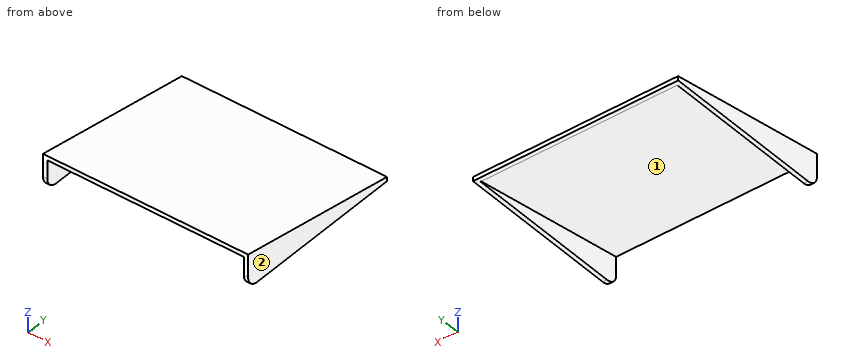
from build123d import *

# Parameters (mm, degrees)
F1_DEPTH = 914.4
F2_T     = -19.05


with BuildPart() as f1:
    # F0 (on Right) → F1 (new body)
    with BuildSketch(Plane.YZ):
        with BuildLine():
            Line((-889, 152.4), (-889, 50.8))
            ThreePointArc((-889, 50.8), (-874.121024, 14.878976), (-838.2, 0))
            Line((-838.2, 0), (-111.125, 0))
            Line((-111.125, 0), (-111.125, 19.05))
            Line((-111.125, 19.05), (-889, 152.4))
        make_face()
    extrude(amount=F1_DEPTH)

    # F2
    f2_openings = [f1.faces().sort_by_distance(p)[0] for p in [
        (457.2, -474.6625, 0),
        (457.2, -874.121024, 14.878976),
        (457.2, -889, 101.6),
    ]]
    offset(amount=F2_T, openings=f2_openings)


solid = f1.part
Geometry check sheet. Reference: the model listing, model coordinates, mm. Face numbers are marked on the shaded views. A direction names the side the tool comes from. Give positions to 0.01 mm unless a question says otherwise; leave off trailing zeros. Loops run counter-clockwise (first coordinate to the right, second up) from the corner with the lowest first, then second, coordinate; pieces in that order, holes last. Notation, with made-up numbers: M 79,1 L 90,1 A15 ccw 90,28 Z; hole C 17,72.25 d8. An arc over 180 degrees is marked long. Write each question's results on one line, items separated by ' | '.
1) Tool access check on the marked faces 1 and 2. Record the directions out of +Z, -Z, +X, -X, +Y, -Y that give a thin tool (end or side, any length) a straight path to the whole face; none if there is none.
Answers follow:
face 1: -Z, -Y | face 2: +Z, -Z, +X, +Y, -Y
2) Section check A-A, the plane y = -773.5. Record the boundary of the cut face in (x, z).
Answers follow:
outline: M 0,0 L 19.05,0 L 19.05,113.27 L 895.35,113.27 L 895.35,0 L 914.4,0 L 914.4,132.6 L 0,132.6 Z
3) Thickness scan on line 1 (X direction, y = -640, z = 16); line 2 (Z direction, x = 411, y = -845); line 3 (Z direction, x = 141, y = -790.5). Record the ranges inside material, lowest first.
Answers follow:
line 1: 0 to 19.05, 895.35 to 914.4 | line 2: 125.53 to 144.86 | line 3: 116.19 to 135.51
4) Section check B-B, the plane z = 78. Record the boundary of the cut face in (x, y), plus the area to 3 significant figures.
Answers follow:
outline: M 0,-889 L 19.05,-889 L 19.05,-567.75 L 895.35,-567.75 L 895.35,-889 L 914.4,-889 L 914.4,-455 L 0,-455 Z | area: 115,000 mm2
5) Section check C-C, the plane x = 565.5. Record the boundary of the cut face in (y, z) (3 decimals).
Answers follow:
outline: M -889,133.072 L -130.175,2.988 L -130.175,0 L -111.125,0 L -111.125,19.05 L -889,152.4 Z
6) Gauge pin test, flat ends, axial feed: pin 1 (5 mm diameter, centred on x = 729.5, y = -782.5, fed in from +Z); pin 2 (3 mm diameter, centred on x = 686, y = -450.5, fed in from +Z); pin 3 (2.5 mm diameter, centred on x = 373, z = 1.5, fed in from -Y) (3 decimals). Record the tip position at first contact, or that the pin passes through.
Answers follow:
pin 1: z = 134.57 | pin 2: z = 77.49 | pin 3: y = -130.175
